```python
from build123d import *

# Parameters (mm, degrees)
F1_DEPTH      = 12.7
F2_R          = 29.3293936748
F3_DEPTH      = 1016
F4_W          = 25.4
F4_H          = 63.5
F5_DEPTH      = 63.5
F7_DEPTH      = 25.4
F7_DEPTH_BACK = 127
F8_R          = 12.7
F9_DEPTH      = 25.4
F9_DEPTH_BACK = 127


with BuildPart() as f1:
    # F0 (on Top) → F1 (new body)
    with BuildSketch(Plane.XY):
        Polygon((-25.4, 105.5293925285), (-25.4, 29.3293925285), (-91.3911340489, -8.7706104496), (-65.9911320635, -52.7646998156), (1.9854e-06, -14.6646968374), (65.9911394732, -52.7646938593), (91.3911374878, -8.7706022007), (25.4, 29.3293948211), (25.4, 105.5293925285), align=None)
    extrude(amount=-F1_DEPTH)

    # F2 (on face) → F3 (join)
    with BuildSketch(Plane.XY):
        with Locations((6.618e-07, 14.6646968374)):
            Circle(F2_R)
    extrude(amount=F3_DEPTH)

    # F4 (on face) → F5 (cut)
    with BuildSketch(Plane.XY.offset(1016)):
        with Locations((6.618e-07, 14.6646968374)):
            Rectangle(F4_W, F4_H)
    extrude(amount=-F5_DEPTH, mode=Mode.SUBTRACT)

    # F6 (on face) → F7 (cut, two sides)
    with BuildSketch(Plane.YZ.offset(-12.6999993382)) as f7_sk:
        Polygon((2.1613299569, 1016), (-11.7724613558, 1016), (-11.7724613558, 994.7630167007), align=None)
    extrude(amount=-F7_DEPTH, mode=Mode.SUBTRACT)
    extrude(f7_sk.sketch, amount=F7_DEPTH_BACK, mode=Mode.SUBTRACT)

    # F8 (on face) → F9 (cut, two sides)
    with BuildSketch(Plane.YZ.offset(-12.6999993382)) as f9_sk:
        with Locations((21.6315924938, 990.6)):
            Circle(F8_R)
    extrude(amount=-F9_DEPTH, mode=Mode.SUBTRACT)
    extrude(f9_sk.sketch, amount=F9_DEPTH_BACK, mode=Mode.SUBTRACT)


solid = f1.part
```
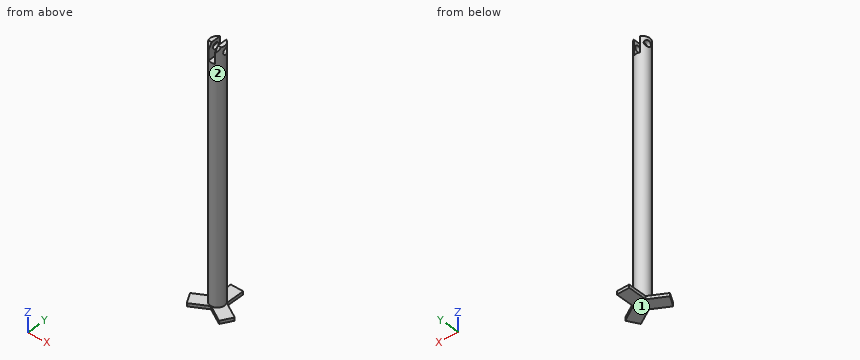
Input: part model. Units: mm. Frame: model coordinates. Face numbers are marked on the shaded views. A direction names the side the tool comes from. Round coordinates to 2 decimals unless told otherwise and drop trailing zeros. Loops run counter-clockwise (first coordinate to the right, second up) from the corner with the lowest first, then second, coordinate; pieces in that order, holes last. Notation, with made-up numbers: (-24, 59.5) -> (25, 59.5) arc R21 cw to (25, 88.5) -> close; hole circle Ø9 at (66.25, 49). An arc over 180 degrees is marked (long way). Write each question's results on one line, items separated by ' | '.
1. Set-up query: the marked faces 1 and 2. Return all of +Z, -Z, +X, -X, +Y, -Y with unobstructed straight access to the full face (end or side cutting, diameter ignored); none if empty.
Geometry results:
face 1: -Z, +X, -X, +Y, -Y | face 2: +Z
2. Section A-A (y = 57.5). Return loops of the section in (x, z), and give its area (3 significant figures).
Geometry results:
outline: (-25.4, -12.7) -> (25.4, -12.7) -> (25.4, 0) -> (-25.4, 0) -> close | area: 645 mm2
3. Ray query, line 1 (Z direction, x = 74, y = -18.5); line 2 (Y direction, x = -19.75, z = 990.6); line 3 (Y direction, x = 17, z = 990). Return the intervals inside material, ascending. Write a range as from..to.
Geometry results:
line 1: -12.7..0 | line 2: -7.02..8.93, 34.33..36.35 | line 3: -9.24..8.95, 34.32..38.56
4. Section B-B (x = 53). Return loops of the section in (y, z).
Geometry results:
outline: (-45.26, -12.7) -> (13.39, -12.7) -> (13.39, 0) -> (-45.26, 0) -> close
5. First-contact query: P1, Ø10, axis at y = 49.5, z = -4, coming from the +X side; P2, Ø4, axis at y = 60, z = -8, coming from the -X side; P3, Ø6, axis at x = 11, y = -2.5, coming from the +Z side; P4, Ø12, axis at x = 29, y = 80.5, coming from the -Z side. Flat tips, straight axial feed; report the tip coordinate or a pass-through.
Geometry results:
P1: x = 25.4 | P2: x = -25.4 | P3: z = 1012.66 | P4: z = -12.7
6. Section C-C (z = 263). Return loops of the section in (x, y), and give its area (3 significant figures).
Geometry results:
outline: circle Ø58.66 at (0, 14.66) | area: 2,700 mm2
